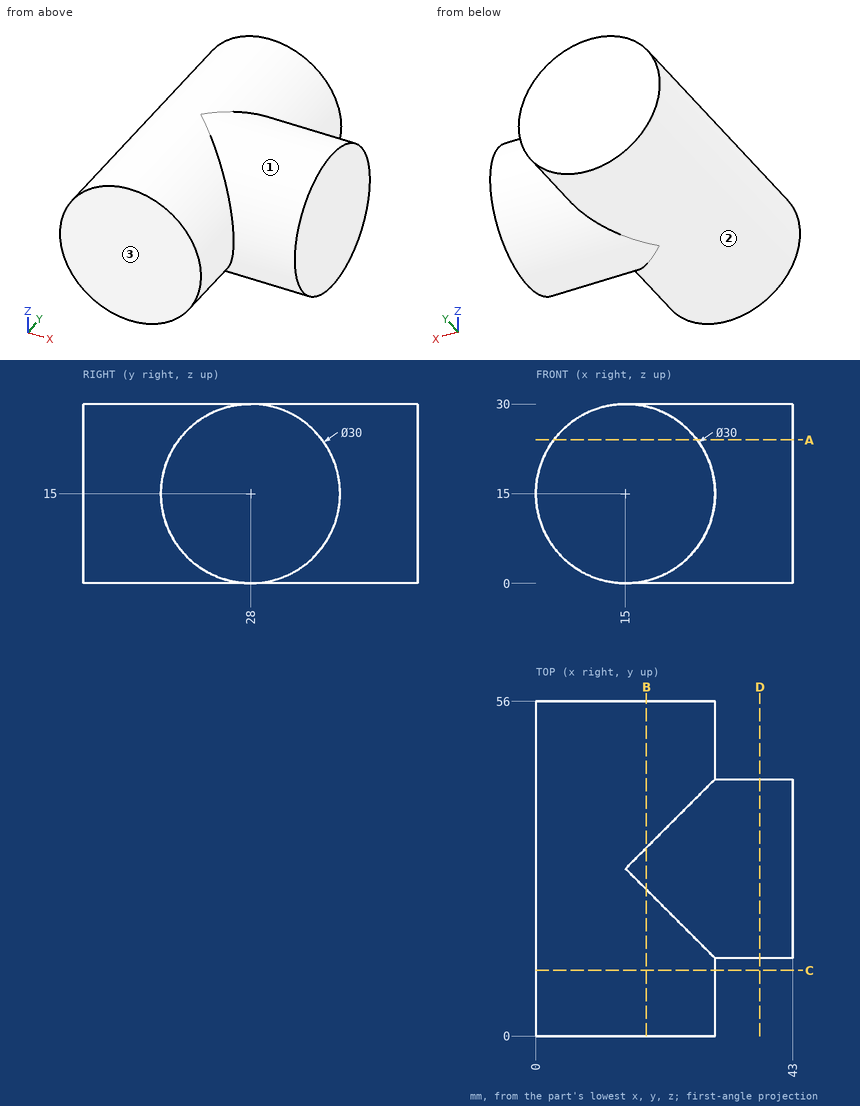
Study the drawing (mm; zero at the part's minimum x, y, z) and answer. A direction names the side the tool comes from. Round coordinates to 2 decimals unless told otherwise and drop trailing zeros. Loops run counter-clockwise (first coordinate to the right, second up) from the corner with the lowest first, then second, coordinate; pieces in that order, holes last. Notation, with made-up numbers: M 87.25,-35 L 144.25,-35 A28 ccw 144.25,3 Z; hole C 34,16 d1. An arc over 180 degrees is marked long. One line per question, with ' | ' between items.
Q1. Consider line 1 along Z through (x, y) = (33, 27.5); line 2 along X through (y, z) = (27, 14.5); line 3 along Z through (x, y) = (7, 42). Determine where each line is inside the solid, lowest interval first. Write a range as from..to.
Conclusion:
line 1: z = 0.01..29.99 | line 2: x = 0.01..43 | line 3: z = 2.31..27.69
Q2. Find section B-B, the plane x = 18.5. Give the vertices of the cut face in (y, z).
Conclusion:
outline: M 0,0.41 L 24.5,0.41 A15 ccw 31.5,0.41 L 56,0.41 L 56,29.59 L 31.5,29.59 A15 ccw 24.5,29.59 L 0,29.59 Z
Q3. Find section C-C, the plane y = 11. Give the vertices of the cut face in (x, z).
Conclusion:
outline: C 15,15 d30
Q4. A tool of negligible diameter and unlimited length cuts with its end or side. For the marked faces 1, 2 and 3, from which of +Z, -Z, +X, -X, +Y, -Y can it reach the whole face along a straight path? Write none if from no direction.
Conclusion:
face 1: +X | face 2: none | face 3: +Z, -Z, +X, -X, -Y
Q5. Each of these flat-tipped pins is pushed along its axis until it touches: pin 1 Ø1.5 at (x, y) = (4.5, 40.5) entering from -Z; pin 2 Ø5 at (x, z) = (16.5, 25.5) entering from -Y; pin 3 Ø5 at (y, z) = (37, 11) entering from -X; pin 4 Ø1.5 at (y, z) = (11, 20) entering from -X. Where does it stop, or does it pass through?
Conclusion:
pin 1: stops at z = 3.6 | pin 2: stops at y = 0 | pin 3: stops at x = 0.08 | pin 4: stops at x = 0.61
Q6. Find section A-A, the plane z = 24. Give the vertices of the cut face in (x, y).
Conclusion:
outline: M 3,0 L 27,0 L 27,16 L 43,16 L 43,40 L 27,40 L 27,56 L 3,56 Z
Q7. Find section D-D, the plane x = 37.5. Give the vertices of the cut face in (y, z).
Conclusion:
outline: C 28,15 d30
